Read the model definition and answer for the solid it produces. Units are mm, in the model's axes. Give positions to 0.01 mm unless a question says otherwise; leave off trailing zeros. Order: outer loops, then holes, each group sorted by start corner. A loop starts at its lowest first (then second) coordinate and runs counter-clockwise, first axis right, second up.
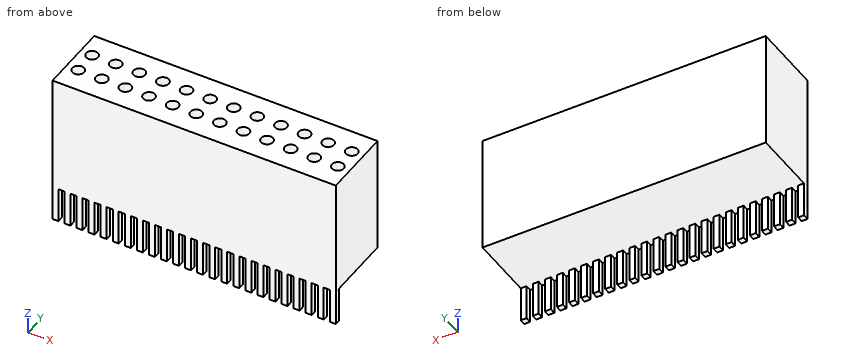
```python
from build123d import *

# Parameters (mm, degrees)
SKETCH2_W           = 24
SKETCH2_H           = 6
BOSS_EXTRUDE1_DEPTH = 10
SKETCH3_R           = 0.5
CUT_EXTRUDE1_DEPTH  = 5
SKETCH4_W           = 0.5
SKETCH4_H           = 3
BOSS_EXTRUDE2_DEPTH = 0.5


with BuildPart() as part:
    # Sketch2 → Boss-Extrude1 (new body)
    with BuildSketch(Plane.XY):
        with Locations((12, 3)):
            Rectangle(SKETCH2_W, SKETCH2_H)
    extrude(amount=BOSS_EXTRUDE1_DEPTH)

    # Sketch3 → Cut-Extrude1 (cut)
    with BuildSketch(Plane.XY.offset(10)):
        with Locations((1, 2)):
            Circle(SKETCH3_R)
        with Locations((3, 2)):
            Circle(SKETCH3_R)
        with Locations((5, 2)):
            Circle(SKETCH3_R)
        with Locations((7, 2)):
            Circle(SKETCH3_R)
        with Locations((9, 2)):
            Circle(SKETCH3_R)
        with Locations((11, 2)):
            Circle(SKETCH3_R)
        with Locations((13, 2)):
            Circle(SKETCH3_R)
        with Locations((15, 2)):
            Circle(SKETCH3_R)
        with Locations((17, 2)):
            Circle(SKETCH3_R)
        with Locations((19, 2)):
            Circle(SKETCH3_R)
        with Locations((21, 2)):
            Circle(SKETCH3_R)
        with Locations((23, 2)):
            Circle(SKETCH3_R)
        with Locations((23, 4)):
            Circle(SKETCH3_R)
        with Locations((21, 4)):
            Circle(SKETCH3_R)
        with Locations((19, 4)):
            Circle(SKETCH3_R)
        with Locations((17, 4)):
            Circle(SKETCH3_R)
        with Locations((15, 4)):
            Circle(SKETCH3_R)
        with Locations((13, 4)):
            Circle(SKETCH3_R)
        with Locations((11, 4)):
            Circle(SKETCH3_R)
        with Locations((9, 4)):
            Circle(SKETCH3_R)
        with Locations((7, 4)):
            Circle(SKETCH3_R)
        with Locations((5, 4)):
            Circle(SKETCH3_R)
        with Locations((3, 4)):
            Circle(SKETCH3_R)
        with Locations((1, 4)):
            Circle(SKETCH3_R)
    extrude(amount=-CUT_EXTRUDE1_DEPTH, mode=Mode.SUBTRACT)

    # Sketch4 → Boss-Extrude2 (add)
    with BuildSketch(Plane(origin=(0, 0, 0), x_dir=(-1, 0, 0), z_dir=(0, -1, 0))):
        with Locations((-0.25, 1.5)):
            Rectangle(SKETCH4_W, SKETCH4_H)
        with Locations((-1.27173914, 1.5)):
            Rectangle(SKETCH4_W, SKETCH4_H)
        with Locations((-2.29347828, 1.5)):
            Rectangle(SKETCH4_W, SKETCH4_H)
        with Locations((-3.31521742, 1.5)):
            Rectangle(SKETCH4_W, SKETCH4_H)
        with Locations((-4.33695656, 1.5)):
            Rectangle(SKETCH4_W, SKETCH4_H)
        with Locations((-5.3586957, 1.5)):
            Rectangle(SKETCH4_W, SKETCH4_H)
        with Locations((-6.38043484, 1.5)):
            Rectangle(SKETCH4_W, SKETCH4_H)
        with Locations((-7.40217398, 1.5)):
            Rectangle(SKETCH4_W, SKETCH4_H)
        with Locations((-8.42391312, 1.5)):
            Rectangle(SKETCH4_W, SKETCH4_H)
        with Locations((-9.44565226, 1.5)):
            Rectangle(SKETCH4_W, SKETCH4_H)
        with Locations((-10.4673914, 1.5)):
            Rectangle(SKETCH4_W, SKETCH4_H)
        with Locations((-11.48913054, 1.5)):
            Rectangle(SKETCH4_W, SKETCH4_H)
        with Locations((-12.51086968, 1.5)):
            Rectangle(SKETCH4_W, SKETCH4_H)
        with Locations((-13.53260882, 1.5)):
            Rectangle(SKETCH4_W, SKETCH4_H)
        with Locations((-14.55434796, 1.5)):
            Rectangle(SKETCH4_W, SKETCH4_H)
        with Locations((-15.5760871, 1.5)):
            Rectangle(SKETCH4_W, SKETCH4_H)
        with Locations((-16.59782624, 1.5)):
            Rectangle(SKETCH4_W, SKETCH4_H)
        with Locations((-17.61956538, 1.5)):
            Rectangle(SKETCH4_W, SKETCH4_H)
        with Locations((-18.64130452, 1.5)):
            Rectangle(SKETCH4_W, SKETCH4_H)
        with Locations((-19.66304366, 1.5)):
            Rectangle(SKETCH4_W, SKETCH4_H)
        with Locations((-20.6847828, 1.5)):
            Rectangle(SKETCH4_W, SKETCH4_H)
        with Locations((-21.70652194, 1.5)):
            Rectangle(SKETCH4_W, SKETCH4_H)
        with Locations((-22.72826108, 1.5)):
            Rectangle(SKETCH4_W, SKETCH4_H)
        with Locations((-23.75000022, 1.5)):
            Rectangle(SKETCH4_W, SKETCH4_H)
    extrude(amount=-BOSS_EXTRUDE2_DEPTH)


solid = part.part
```
1) Consider L1, parallel to Y at x = 21, z = 7.75; L2, parallel to Y at x = 17.5, z = -1; L3, parallel to Z at x = 2.75, y = 1.35. Determine where each line is inside the solid, lowest interval first.
Final values:
L1: y = 0 to 1.5, 2.5 to 3.5, 4.5 to 6
L2: y = 0 to 0.5
L3: z = 0 to 10
2) The part is cut by section A-A on z = 5.5. Count the separate pieces of the cut face and the enclosed holes in it, and give its area (3 significant figures).
Final values:
separate pieces: 1
enclosed holes: 24
area: 125 mm2
3) The part is cut by section C-C on y = 5.6. Determine the outline of the cut face in (x, z), and give its area (3 significant figures).
Final values:
outline: (0, 0) - (24, 0) - (24, 10) - (0, 10) - close
area: 240 mm2
4) Given pin 1 (0.5 mm diameter, centred on x = 13, y = 2, fed in from +Z); pin 2 (0.6 mm diameter, centred on y = 0.5, z = -1.5, fed in from -X), each flat-ended and moving along its own axis, determine where each tip first touches the part or whether it passes through.
Final values:
pin 1: stops at z = 5
pin 2: stops at x = 0
5) The part is cut by section B-B on x = 11. Determine the outline of the cut face in (y, z).
Final values:
outline: (0, 0) - (6, 0) - (6, 10) - (4.5, 10) - (4.5, 5) - (3.5, 5) - (3.5, 10) - (2.5, 10) - (2.5, 5) - (1.5, 5) - (1.5, 10) - (0, 10) - close
